Job drawing, mm, ordinate dimensions from the low corner. One solid piece. Give positions to 0.01 mm unless a question says otherwise; leave off trailing zeros. Order: outer loops, then holes, each group sorted by start corner. A loop starts at its lowest first (then second) coordinate and runs counter-clockwise, first axis right, second up.
1. Slice it at A-A on y = 35.56. List the corners of the cut face in (x, z).
2. Drop flat-ended pins along their axis: pin 1 Ø5 at (x, z) = (64, 10.5) entering from -Y (1 decimal); pin 2 Ø3.5 at (x, z) = (38.1, 6.35) entering from +Y; pin 3 Ø3 at (x, z) = (7.62, 6.35) entering from -Y. Give the stop position or say it passes through.
3. Mould opens along Y. For the marked faces 1, 2 and 3 say: +Y half, -Y half, draft (parallel to the pull), parting line (faces both ways), or undercut.
4. Slice it at D-D on z = 3. Give the number of separate pieces and of enclosed holes in the cut face, and give its area (3 significant figures).
5. Slice it at B-B on y = 22.86. List the corners of the cut face in (x, z).
6. Probe line 1 (X direction, y = 45, z = 6.25) (1 decimal); line 2 (X direction, y = 23, z = 3); line 3 (Z direction, x = 38.1, y = 45.5). List the from-to ranges inside material, lowest first.
7. Slice it at C-C on x = 55.5. List the corners of the cut face in (y, z) (1 decimal), and give its area (3 significant figures).
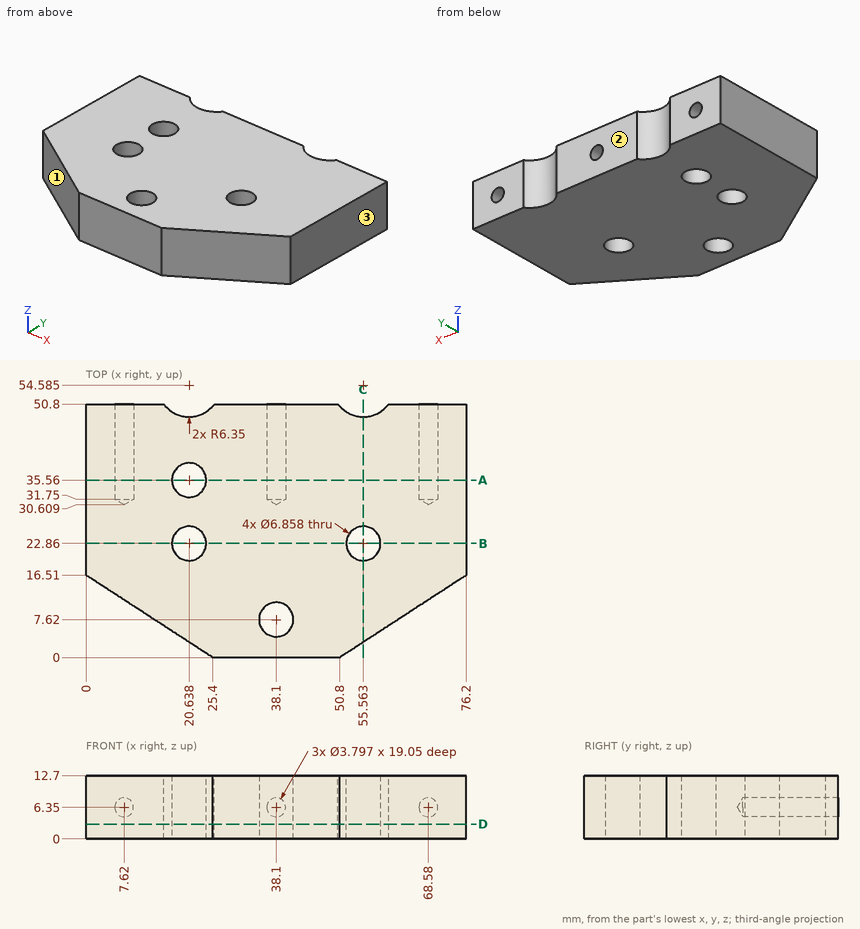
Data:
1. outline: (0, 0) - (17.21, 0) - (17.21, 12.7) - (0, 12.7) - close; (24.07, 0) - (76.2, 0) - (76.2, 12.7) - (24.07, 12.7) - close; hole circle Ø3.8 at (7.62, 6.35); hole circle Ø3.8 at (38.1, 6.35); hole circle Ø3.8 at (68.58, 6.35)
2. pin 1: stops at y = 7
2. pin 2: stops at y = 31.66
2. pin 3: stops at y = 10.58
3. face 1: -Y half
3. face 2: +Y half
3. face 3: draft
4. separate pieces: 1
4. enclosed holes: 4
4. area: 3,270 mm2
5. outline: (0, 0) - (17.21, 0) - (17.21, 12.7) - (0, 12.7) - close; (24.07, 0) - (52.13, 0) - (52.13, 12.7) - (24.07, 12.7) - close; (58.99, 0) - (76.2, 0) - (76.2, 12.7) - (58.99, 12.7) - close
6. line 1: x = 0 to 5.7, 9.5 to 36.2, 40 to 66.7, 70.5 to 76.2
6. line 2: x = 0 to 17.21, 24.06 to 52.14, 58.99 to 76.2
6. line 3: z = 0 to 4.45, 8.25 to 12.7
7. outline: (3.1, 0) - (19.4, 0) - (19.4, 12.7) - (3.1, 12.7) - close; (26.3, 0) - (48.2, 0) - (48.2, 12.7) - (26.3, 12.7) - close
7. area: 487 mm2
